from build123d import *

# Parameters (mm, degrees)
SKETCH1_R           = 6
EXTRUDE1_DEPTH      = 100
CHAMFER1_SIZE       = 0.9
EXTRUDE3_DEPTH      = 101.359354322
EXTRUDE3_DEPTH_BACK = 101.359354322
SKETCH2_R           = 2


with BuildPart() as part:
    # Sketch1 → Extrude1 (new, symmetric)
    with BuildSketch(Plane.XY):
        Circle(SKETCH1_R)
    extrude(amount=EXTRUDE1_DEPTH, both=True)

    # Chamfer1
    chamfer1_edges = [part.edges().sort_by_distance(p)[0] for p in [
        (-6, 0, -100),
    ]]
    chamfer(chamfer1_edges, length=CHAMFER1_SIZE)

    # Sketch2 → Extrude3 (cut, two sides: drawn at the far end of the back side and taken through both)
    with BuildSketch(Plane.XY.offset(-EXTRUDE3_DEPTH_BACK)):
        Circle(SKETCH2_R)
    extrude(amount=EXTRUDE3_DEPTH + EXTRUDE3_DEPTH_BACK, mode=Mode.SUBTRACT)

    # Sketch5 → Groove for DIN 471 - 12 x 1_ Circlip for (revolve, cut)
    with BuildSketch(Plane(origin=(0, 0, 100), x_dir=(0, 1, 0), z_dir=(-1, 0, 0)), mode=Mode.PRIVATE) as groove_for_din_471_12_x_1_circlip_for_sk:
        with BuildLine():
            Line((5.86, 61.5), (7.2, 61.5))
            Line((7.2, 61.5), (7.2, 62.6))
            Line((7.2, 62.6), (5.86, 62.6))
            ThreePointArc((5.86, 62.6), (5.782218254, 62.567781746), (5.75, 62.49))
            Line((5.75, 62.49), (5.75, 61.61))
            ThreePointArc((5.75, 61.61), (5.782218254, 61.532218254), (5.86, 61.5))
        make_face()
    revolve(groove_for_din_471_12_x_1_circlip_for_sk.sketch.rotate(Axis((0, 0, 150), (0, 0, -1)), 270), axis=Axis((0, 0, 150), (0, 0, -1)), mode=Mode.SUBTRACT)

    # Sketch13 → Groove for DIN 471 - 12 x 1_ Circlip 2 (revolve, cut)
    with BuildSketch(Plane(origin=(0, 0, 100), x_dir=(0, 1, 0), z_dir=(-1, 0, 0)), mode=Mode.PRIVATE) as groove_for_din_471_12_x_1_circlip_2_sk:
        with BuildLine():
            Line((5.86, 174.7), (7.2, 174.7))
            Line((7.2, 174.7), (7.2, 175.8))
            Line((7.2, 175.8), (5.86, 175.8))
            ThreePointArc((5.86, 175.8), (5.782218254, 175.767781746), (5.75, 175.69))
            Line((5.75, 175.69), (5.75, 174.81))
            ThreePointArc((5.75, 174.81), (5.782218254, 174.732218254), (5.86, 174.7))
        make_face()
    revolve(groove_for_din_471_12_x_1_circlip_2_sk.sketch.rotate(Axis((0, 0, 150), (0, 0, -1)), 270), axis=Axis((0, 0, 150), (0, 0, -1)), mode=Mode.SUBTRACT)


solid = part.part
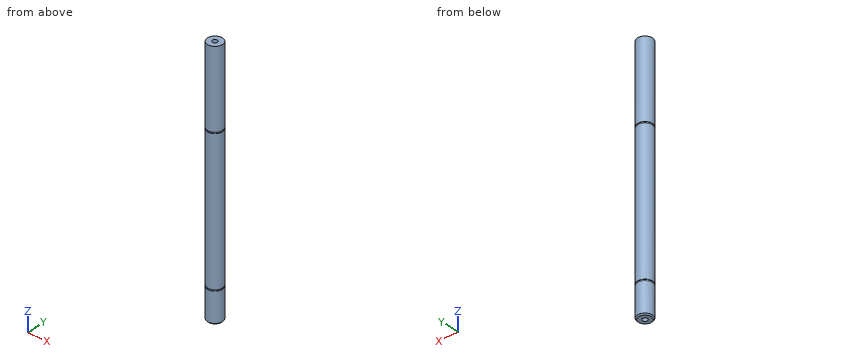
Source: CAD feature listing. Evaluate the final solid. Frame: model axes, mm. Round coordinates to 2 decimals unless told otherwise and drop trailing zeros. Loops run counter-clockwise (first coordinate to the right, second up) from the corner with the lowest first, then second, coordinate; pieces in that order, holes last. Notation, with made-up numbers: (-19.75, 24.5) - (18.25, 24.5) arc R19 cw to (18.25, 36.5) - close; hole circle Ø5 at (-5, -31.5). An arc over 180 degrees is marked (long way). Write item = value, one per line. Start each with the question number.
(1) Section query C-C, the plane z = -36. Output: boundary loops of the cut face in (x, y).
(2) Ray query, line 1 along Y through (x, z) = (0, -19.5); line 2 along Z through (x, y) = (-5, 3); line 3 along X through (y, z) = (1.75, 44). Return the intervals inside material, ascending. Write a range as from..to.
(3) Pin query (flat end, axial travel): pin 1 (3 mm diameter, centred on y = 3, z = -68.5, fed in from +X); pin 2 (3.5 mm diameter, centred on x = 0, y = 0, fed in from +Z); pin 3 (6 mm diameter, centred on y = -3.5, z = 7.5, fed in from +X). Return the tip coordinate at first contact, or that it passes through.
Conclusion:
q1.outline = circle Ø12 at (0, 0); hole circle Ø4 at (0, 0)
q2.line_1 = -6..-2, 2..6
q2.line_2 = -99.27..-75.8, -74.7..37.4, 38.5..100
q2.line_3 = -5.74..-0.97, 0.97..5.74
q3.pin_1 = 5.81
q3.pin_2 = through
q3.pin_3 = 5.98
